```python
from build123d import *

# Parameters (mm, degrees)
BOSS_EXTRUDE1_DEPTH = 1.524


with BuildPart() as part:
    # Sketch1 → Boss-Extrude1 (new body)
    with BuildSketch(Plane.XY):
        with BuildLine():
            Line((1.524, 26.967680282), (0, 26.967680282))
            Line((0, 26.967680282), (0, 22.217880282))
            Line((0, 22.217880282), (1.524, 22.217880282))
            Line((1.524, 22.217880282), (1.524, 18.391271339))
            ThreePointArc((1.524, 18.391271339), (2.358852733, 18.057327031), (3.193705465, 18.391271339))
            Line((3.193705465, 18.391271339), (3.241105721, 20.110110457))
            ThreePointArc((3.241105721, 20.110110457), (5.645287311, 19.111172108), (8.181482071, 19.699120308))
            Line((8.181482071, 19.699120308), (10.646545317, 21.491818606))
            Line((10.646545317, 21.491818606), (7.781599903, 25.431283294))
            Line((7.781599903, 25.431283294), (5.316536657, 23.638584995))
            ThreePointArc((5.316536657, 23.638584995), (4.31894521, 23.329334303), (3.339913307, 23.693094141))
            Line((3.339913307, 23.693094141), (3.378365348, 25.087450992))
            ThreePointArc((3.378365348, 25.087450992), (2.095759725, 27.920506851), (1.524, 30.977363652))
            Line((1.524, 30.977363652), (1.524, 26.967680282))
        make_face()
    extrude(amount=BOSS_EXTRUDE1_DEPTH)


solid = part.part
```
Geometry check sheet. Reference: the model listing, model coordinates, mm. A direction names the side the tool comes from. Round coordinates to 2 decimals unless told otherwise and drop trailing zeros. Order: outer loops, then holes, each group sorted by start corner. A loop starts at its lowest first (then second) coordinate and runs counter-clockwise, first axis right, second up. Notation, with made-up numbers: (72, 46) -> (129, 46) arc R23 cw to (129, 71) -> close; hole circle Ø9 at (17.5, -12.5). An arc over 180 degrees is marked (long way). Return JSON: item names as keys, results as strings. Group by question number.
Q1. Section check A-A, the plane z = 1.15. Record the boundary of the cut face in (x, y).
Q2. Section check C-C, the plane x = 6.5. Record the boundary of the cut face in (y, z).
Q3. Material ranges on probe 1 along Y at (x, z) = (1.25, 1.2); probe 2 along X at (y, z) = (18.5, 0.8); probe 3 along X at (y, z) = (24.5, 0.7), recorded low to high. Write a range as from..to.
Q4. Release check for a two-part mould opening along X. For faces 4 (the flat face through (4, 23, 1.524)), 5 (the cylindrical face through (4.33, 23.33, 0.75)), 6 (the flat face through (9.397, 20.583, 0.751)), 7 (the cylindrical face through (5.608, 19.114, 0.751)) record: released by +X, released by -X, zero draft, split by the parting line, or undercut.
Q5. Section check B-B, the plane y = 24.5. Record the boundary of the cut face in (x, z).
Q6. Gauge pin test, flat ends, axial feed: pin 1 (0.8 mm diameter, centred on y = 29, z = 0.5, fed in from -X); pin 2 (0.8 mm diameter, centred on x = 0.5, z = 0.5, fed in from +Y); pin 3 (0.8 mm diameter, centred on x = 1, z = 0.5, fed in from -Y). Record the tip position at first contact, or that the pin passes through.
Q7. Tool access check on faces 1 (the flat face through (6.57, 24.55, 0.75)), 2 (the flat face through (1.524, 29, 1)), 3 (the flat face through (1.524, 20, 1)). Record the directions out of +Z, -Z, +X, -X, +Y, -Y that give a thin tool (end or side, any length) a straight path to the whole face; none if there is none.
Q8. Section check D-D, the plane y = 26.75. Record the boundary of the cut face in (x, z), plus the area to 3 significant figures.
Numbers:
{
 "1": {"outline": "(0, 22.22) -> (1.52, 22.22) -> (1.52, 18.39) arc R1.21 ccw to (3.19, 18.39) -> (3.24, 20.11) arc R4.26 ccw to (8.18, 19.7) -> (10.65, 21.49) -> (7.78, 25.43) -> (5.32, 23.64) arc R1.62 cw to (3.34, 23.69) -> (3.38, 25.09) arc R12.98 cw to (1.52, 30.98) -> (1.52, 26.97) -> (0, 26.97) -> close"},
 "2": {"outline": "(19.13, 0) -> (24.5, 0) -> (24.5, 1.52) -> (19.13, 1.52) -> close"},
 "3": {"probe 1": "22.22..26.97", "probe 2": "1.52..3.2", "probe 3": "0..3.36, 6.5..8.46"},
 "4": {"face 4": "zero draft", "face 5": "undercut", "face 6": "released by +X", "face 7": "undercut"},
 "5": {"outline": "(0, 0) -> (3.36, 0) -> (3.36, 1.52) -> (0, 1.52) -> close; (6.5, 0) -> (8.46, 0) -> (8.46, 1.52) -> (6.5, 1.52) -> close"},
 "6": {"pin 1": "x = 1.52", "pin 2": "y = 26.97", "pin 3": "y = 22.22"},
 "7": {"face 1": "+Z, -Z, +Y", "face 2": "+Z, -Z, -X, +Y", "face 3": "+Z, -Z, -X, -Y"},
 "8": {"outline": "(0, 0) -> (2.53, 0) -> (2.53, 1.52) -> (0, 1.52) -> close", "area": "3.85 mm^2"}
}
